The listing builds one solid part. Answer for the finished solid, in the listing's coordinates (mm). A direction names the side the tool comes from. Give positions to 0.01 mm unless a question says otherwise; leave off trailing zeros. Write each loop counter-clockwise with the first axis right and the second up, starting at its lowest first coordinate (ties: lowest second). Pieces come first, ordered by that corner, then holes. Notation, with made-up numbers: (55, -39.75) - (72, -39.75) arc R24 cw to (72, -0.75) - close; hole circle Ø11 at (-4.5, 15). An arc over 180 degrees is marked (long way). Answer in a Markdown table with one row per item. Add a question column.
from build123d import *

# Parameters (mm, degrees)
SKETCH1_R           = 125
SKETCH1_R_2         = 4
BOSS_EXTRUDE1_DEPTH = 25
SKETCH4_R           = 9
CUT_EXTRUDE1_DEPTH  = 10
SKETCH6_R           = 5
CUT_EXTRUDE2_DEPTH  = 15
SKETCH7_R           = 50
CUT_EXTRUDE3_DEPTH  = 3
SKETCH8_R           = 105
SKETCH8_R_2         = 85
BOSS_EXTRUDE2_DEPTH = 10


with BuildPart() as part:
    # Sketch1 → Boss-Extrude1 (new body)
    with BuildSketch(Plane(origin=(0, 0, 0), x_dir=(1, 0, 0), z_dir=(0, 1, 0))):
        Circle(SKETCH1_R)
        with Locations((0, 115)):
            Circle(SKETCH1_R_2, mode=Mode.SUBTRACT)
        with Locations((99.592921435, 57.5)):
            Circle(SKETCH1_R_2, mode=Mode.SUBTRACT)
        with Locations((99.592921435, -57.5)):
            Circle(SKETCH1_R_2, mode=Mode.SUBTRACT)
        with Locations((0, -115)):
            Circle(SKETCH1_R_2, mode=Mode.SUBTRACT)
        with Locations((-99.592921435, -57.5)):
            Circle(SKETCH1_R_2, mode=Mode.SUBTRACT)
        with Locations((-99.592921435, 57.5)):
            Circle(SKETCH1_R_2, mode=Mode.SUBTRACT)
    extrude(amount=BOSS_EXTRUDE1_DEPTH)

    # Sketch4 → Cut-Extrude1 (cut)
    with BuildSketch(Plane.XZ):
        with Locations((-24.748737342, 24.748737342)):
            Circle(SKETCH4_R)
        with Locations((24.748737342, 24.748737342)):
            Circle(SKETCH4_R)
        with Locations((24.748737342, -24.748737342)):
            Circle(SKETCH4_R)
        with Locations((-24.748737342, -24.748737342)):
            Circle(SKETCH4_R)
    extrude(amount=-CUT_EXTRUDE1_DEPTH, mode=Mode.SUBTRACT)

    # Sketch6 → Cut-Extrude2 (cut)
    with BuildSketch(Plane.XZ.offset(-10)):
        with Locations((-24.748737342, 24.748737342)):
            Circle(SKETCH6_R)
        with Locations((24.748737342, 24.748737342)):
            Circle(SKETCH6_R)
        with Locations((24.748737342, -24.748737342)):
            Circle(SKETCH6_R)
        with Locations((-24.748737342, -24.748737342)):
            Circle(SKETCH6_R)
    extrude(amount=-CUT_EXTRUDE2_DEPTH, mode=Mode.SUBTRACT)

    # Sketch7 → Cut-Extrude3 (cut)
    with BuildSketch(Plane(origin=(0, 25, 0), x_dir=(1, 0, 0), z_dir=(0, 1, 0))):
        Circle(SKETCH7_R)
    extrude(amount=-CUT_EXTRUDE3_DEPTH, mode=Mode.SUBTRACT)

    # Sketch8 → Boss-Extrude2 (add)
    with BuildSketch(Plane(origin=(0, 25, 0), x_dir=(1, 0, 0), z_dir=(0, 1, 0))):
        Circle(SKETCH8_R)
        Circle(SKETCH8_R_2, mode=Mode.SUBTRACT)
    extrude(amount=BOSS_EXTRUDE2_DEPTH)


solid = part.part
1. A tool of negligible diameter and unlimited length cuts with its end or side. For faces 5 (the face through (-19.98, 15.92, -23.25)), 6 (the face through (29.587, 4.93, 32.338)), 7 (the face through (-28.4, 25, 101.3)), from which of +Z, -Z, +X, -X, +Y, -Y can it reach the whole face along a straight path? Write none if from no direction.
2. Section A-A (x = 0) is taken. Give the vertices of the cut face in (y, z), and give its area (3 significant figures).
3. Given pin 1 Ø3 at (x, y) = (-41, 22) entering from -Z; pin 2 Ø2 at (y, z) = (13, -85) entering from +X; pin 3 Ø5 at (y, z) = (16, -88.5) entering from +X; pin 4 Ø7 at (x, z) = (0, 115) entering from -Y, each flat-ended and moving along its own axis, determine where each tip first touches the part or whether it passes through.
4. Section D-D (y = 16.5) is taken. State how many separate pieces and enclosed holes the cut face has, and give its area (3 significant figures).
5. Section B-B (z = 0) is taken. Give the vertices of the cut face in (x, y), and give its area (3 significant figures).
6. Section C-C (z = -115) is taken. Give the vertices of the cut face in (x, y), and give its area (3 significant figures).
7. Straight lines are drawn through the part: L1, parallel to Z at x = 0, y = 22.95; L2, parallel to Z at x = 0, y = 6; L3, parallel to X at y = 14.5, z = 59. For each, find the intervals that lie inside material, in ascending order. Write a range as [from, to].
8. The mould has two halves that part along Z. Classify faces 1 (the face through (-0.521, 12.325, 111.034)), 2 (the face through (-8, 35, 85)), 3 (the face through (33.333, 4.93, -22.045)), 4 (the face through (100.15, 29.93, -31.54)): +Z half, -Z half, draft (parallel to the pull), parting line (faces both ways), or undercut.
Geometry check:
| question | item | result |
|---|---|---|
| 1 | face 5 | +Y, -Y |
| 1 | face 6 | -Y |
| 1 | face 7 | +Y |
| 2 | outline | (0, -125) - (25, -125) - (25, -119) - (0, -119) - close; (0, -111) - (25, -111) - (25, -105) - (35, -105) - (35, -85) - (25, -85) - (25, -50) - (22, -50) - (22, 50) - (25, 50) - (25, 85) - (35, 85) - (35, 105) - (25, 105) - (25, 111) - (0, 111) - close; (0, 119) - (25, 119) - (25, 125) - (0, 125) - close |
| 2 | area | 5,950 mm² |
| 3 | pin 1 | z = -118.59 |
| 3 | pin 2 | x = 92.57 |
| 3 | pin 3 | x = 90.71 |
| 3 | pin 4 | through |
| 4 | separate pieces | 1 |
| 4 | enclosed holes | 10 |
| 4 | area | 48,500 mm² |
| 5 | outline | (-125, 0) - (125, 0) - (125, 25) - (105, 25) - (105, 35) - (85, 35) - (85, 25) - (50, 25) - (50, 22) - (-50, 22) - (-50, 25) - (-85, 25) - (-85, 35) - (-105, 35) - (-105, 25) - (-125, 25) - close |
| 5 | area | 6,350 mm² |
| 6 | outline | (-48.99, 0) - (-4, 0) - (-4, 25) - (-48.99, 25) - close; (4, 0) - (48.99, 0) - (48.99, 25) - (4, 25) - close |
| 6 | area | 2,250 mm² |
| 7 | L1 | [-125, -119], [-111, -50], [50, 111], [119, 125] |
| 7 | L2 | [-125, -119], [-111, 111], [119, 125] |
| 7 | L3 | [-110.2, -103.3], [-95.88, 95.88], [103.3, 110.2] |
| 8 | face 1 | undercut |
| 8 | face 2 | draft |
| 8 | face 3 | undercut |
| 8 | face 4 | parting line |
